from build123d import *

# Parameters (mm, degrees)
PAD_DEPTH   = 10
FILLET_R    = 0.8
FILLET001_R = 0.8


with BuildPart() as part:
    # Sketch → Pad (new body)
    with BuildSketch(Plane.XY):
        Polygon((5.7, -5.85), (5.7, -4), (1.5, -4), (1.5, 4), (5.7, 4), (5.7, 5.85), (4.5, 5.5), (1.5, 5.5), (1.5, 6.5), (0, 6.5), (0, -6.5), (1.5, -6.5), (1.5, -5.5), (4.5, -5.5), align=None)
    extrude(amount=PAD_DEPTH)

    # Fillet
    fillet_edges = [part.edges().sort_by_distance(p)[0] for p in [
        (0, 6.5, 5),
        (0, -6.5, 5),
    ]]
    fillet(fillet_edges, radius=FILLET_R)

    # Fillet001
    fillet001_edges = [part.edges().sort_by_distance(p)[0] for p in [
        (5.7, 4, 5),
        (5.7, -4, 5),
    ]]
    fillet(fillet001_edges, radius=FILLET001_R)


solid = part.part
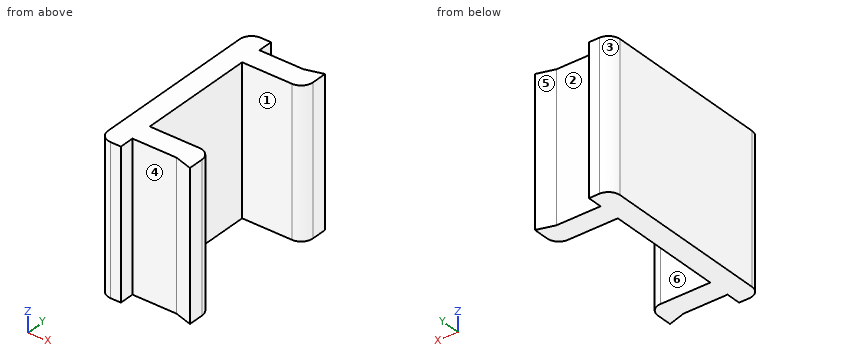
The listing builds one solid part. Answer for the finished solid, in the listing's coordinates (mm). Face numbers are marked on the shaded views. A direction names the side the tool comes from. Round coordinates to 2 decimals unless told otherwise and drop trailing zeros. Order: outer loops, then holes, each group sorted by start corner. A loop starts at its lowest first (then second) coordinate and runs counter-clockwise, first axis right, second up. Notation, with made-up numbers: (82.25, 61.25) -> (95.25, 61.25) arc R29 ccw to (95.25, 94.25) -> close; hole circle Ø1 at (74, 66.25). An arc over 180 degrees is marked (long way). Write each question's results on one line, items separated by ' | '. Start each with the question number.
Q1. Find section C-C (y = -1). Determine the outline of the cut face in (x, z).
Q2. Each of these flat-tipped pins is pushed along its axis until it touches: pin 1 (6 mm diameter, centred on y = -1.5, z = 1.5, fed in from +X); pin 2 (2 mm diameter, centred on x = 4, z = 7.5, fed in from -Y); pin 3 (4 mm diameter, centred on y = -0.5, z = 7.5, fed in from +X). Where does it stop, or does it pass through?
Q3. Find section D-D (y = 4.25). Determine the outline of the cut face in (x, z), then the cut area to 3 significant figures.
Q4. Find section B-B (z = 1.5). Determine the outline of the cut face in (x, y), then the cut area to 3 significant figures.
Q5. Which of the six approach directions +Z, -Z, +X, -X, +Y, -Y give full straight-line access (tool end or side, diameter ignored) to the marked faces 1, 2 and 3?
Q6. Straight lines are drawn through the part: probe 1 along Y at (x, z) = (1.9, 7); probe 2 along X at (y, z) = (-3, 6.5); probe 3 along X at (y, z) = (-4.75, 6.5). For each, find the intervals that lie inside material, in ascending order. Write a range as from..to.
Q7. Find section A-A (x = 2.3). Determine the outline of the cut face in (y, z), then the cut area to 3 significant figures.
Q8. The mould has two halves that part along Y. Classify the marked faces 4, 5 and 6: pulls with the +Y half, pulls with the -Y half, needs draft (parallel to the pull), parting line crosses it, or undercut.
Worked answers:
1) outline: (0, 0) -> (1.5, 0) -> (1.5, 10) -> (0, 10) -> close
2) pin 1: stops at x = 5.64 | pin 2: stops at y = -5.65 | pin 3: stops at x = 1.5
3) outline: (0, 0) -> (5.48, 0) -> (5.48, 10) -> (0, 10) -> close | area: 54.8 mm2
4) outline: (0, -5.7) arc R0.8 ccw to (0.8, -6.5) -> (1.5, -6.5) -> (1.5, -5.5) -> (4.5, -5.5) -> (5.7, -5.85) -> (5.7, -4.8) arc R0.8 ccw to (4.9, -4) -> (1.5, -4) -> (1.5, 4) -> (4.9, 4) arc R0.8 ccw to (5.7, 4.8) -> (5.7, 5.85) -> (4.5, 5.5) -> (1.5, 5.5) -> (1.5, 6.5) -> (0.8, 6.5) arc R0.8 ccw to (0, 5.7) -> close | area: 32.0 mm2
5) face 1: +Z, -Z, +X | face 2: +Z, -Z, +Y | face 3: +Z, -Z, -X, +Y
6) probe 1: y = -5.5..-4, 4..5.5 | probe 2: x = 0..1.5 | probe 3: x = 0..5.7
7) outline: (-5.5, 0) -> (-4, 0) -> (-4, 10) -> (-5.5, 10) -> close; (4, 0) -> (5.5, 0) -> (5.5, 10) -> (4, 10) -> close | area: 30.0 mm2
8) face 4: pulls with the -Y half | face 5: pulls with the +Y half | face 6: undercut
